Build history of the part. All positions in model axes, mm. A direction names the side the tool comes from. Give positions to 0.01 mm unless a question says otherwise; leave off trailing zeros. Order: outer loops, then holes, each group sorted by start corner. A loop starts at its lowest first (then second) coordinate and runs counter-clockwise, first axis right, second up. Notation, with made-up numbers: (5, 49.25) - (14, 49.25) arc R11 ccw to (14, 54.25) - close; hole circle Ø6 at (85.5, -39.5). An arc over 180 degrees is marked (long way). Use a Markdown table: item, result. Add a question column.
(1) Slice it at A-A (y = 6). Write the cut outline in (x, z).
(2) Flat gauge pins, fed straight in: pin 1 (15 mm diameter, centred on x = -20, z = 1.5, fed in from +Y); pin 2 (6 mm diameter, centred on y = 36.5, z = 20.5, fed in from -X); pin 3 (12 mm diameter, centred on x = -31, y = 32, fed in from +Z). Where does each tip first touch, or does it go through?
(3) Slice it at B-B (x = 0). Write the cut outline in (y, z), then the cut area to 3 significant figures.
(4) Slice it at C-C (y = 60). Write the cut outline in (x, z).
(5) Slice it at D-D (z = 21.5). Write the cut outline in (x, y), then the cut area to 3 significant figures.
(6) Wall check: line 1 (X direction, y = 5.5, z = -4.5); line 2 (Z direction, x = 30, y = 4); line 3 (Y direction, x = -0.5, z = 8). Give the ranges that are in metal, low to high.
(7) Which spindle directions (+Z, -Z, +X, -X, +Y, -Y) get a long thin tool onto all of the face, cutting with end or side? Do faces 1 (the face through (45.49, 5.07, -15.72)), 2 (the face through (-1, 10, -5)). Say none if no direction does.
(8) Mould opens along Z. For faces 3 (the face through (1, 38, 10)), 4 (the face through (50, 5, 8)), 5 (the face through (-25.105, 4.92, -5.215)) say: +Z half, -Z half, draft (parallel to the pull), parting line (faces both ways), or undercut.
from build123d import *

# Parameters (mm, degrees)
CROQUIS1_W                           = 100
CROQUIS1_H                           = 40
SALIENTE_EXTRUIR1_DEPTH              = 10
CROQUIS2_R                           = 8
SALIENTE_EXTRUIR2_DEPTH              = 10
SALIENTE_EXTRUIR3_START              = 5
CROQUIS3_R                           = 20
CROQUIS3_R_2                         = 8
SALIENTE_EXTRUIR3_DEPTH              = 5
F_9_8_9_8_DIAMETER_HOLE1_D           = 9.8
F_9_8_9_8_DIAMETER_HOLE1_CSINK_D     = 9.85
F_9_8_9_8_DIAMETER_HOLE1_CSINK_ANGLE = 100
F_10_0_10_DIAMETER_HOLE1_D           = 10
F_10_0_10_DIAMETER_HOLE1_CSINK_D     = 10.05
F_10_0_10_DIAMETER_HOLE1_CSINK_ANGLE = 100
REDONDEO1_R                          = 15


with BuildPart() as part:
    # Croquis1 → Saliente-Extruir1 (new body)
    with BuildSketch(Plane(origin=(0, 0, 0), x_dir=(1, 0, 0), z_dir=(0, 1, 0))):
        Rectangle(CROQUIS1_W, CROQUIS1_H)
    extrude(amount=SALIENTE_EXTRUIR1_DEPTH)

    # Croquis2 → Saliente-Extruir2 (add)
    with BuildSketch(Plane.XY.offset(20)):
        with BuildLine():
            Line((-50, 10), (-17.564659966, 69.564659966))
            ThreePointArc((-17.564659966, 69.564659966), (0, 80), (17.564659966, 69.564659966))
            Line((17.564659966, 69.564659966), (50, 10))
            Line((50, 10), (-50, 10))
        make_face()
        with Locations((0, 60)):
            Circle(CROQUIS2_R, mode=Mode.SUBTRACT)
    extrude(amount=-SALIENTE_EXTRUIR2_DEPTH)

    # Croquis3 → Saliente-Extruir3 (add)
    with BuildSketch(Plane.XY.offset(20).offset(SALIENTE_EXTRUIR3_START)):
        with Locations((0, 60)):
            Circle(CROQUIS3_R)
        with Locations((0, 60)):
            Circle(CROQUIS3_R_2, mode=Mode.SUBTRACT)
    extrude(amount=-SALIENTE_EXTRUIR3_DEPTH)

    # Ø9.8 (9.8) Diameter Hole1 (through all)
    with Locations(Plane(origin=(0, 10, 0), x_dir=(1, 0, 0), z_dir=(0, 1, 0))):
        with Locations((-30, 5)):
            CounterSinkHole(F_9_8_9_8_DIAMETER_HOLE1_D / 2, F_9_8_9_8_DIAMETER_HOLE1_CSINK_D / 2, counter_sink_angle=F_9_8_9_8_DIAMETER_HOLE1_CSINK_ANGLE)

    # Ø10.0 (10) Diameter Hole1 (through all)
    with Locations(Plane(origin=(0, 10, 0), x_dir=(1, 0, 0), z_dir=(0, 1, 0))):
        with Locations((30, 5)):
            CounterSinkHole(F_10_0_10_DIAMETER_HOLE1_D / 2, F_10_0_10_DIAMETER_HOLE1_CSINK_D / 2, counter_sink_angle=F_10_0_10_DIAMETER_HOLE1_CSINK_ANGLE)

    # Redondeo1
    redondeo1_edges = [part.edges().sort_by_distance(p)[0] for p in [
        (-50, 5, -20),
        (50, 5, -20),
    ]]
    fillet(redondeo1_edges, radius=REDONDEO1_R)


solid = part.part
Solution:
| question | item | result |
|---|---|---|
| 1 | outline | (-50, -5) arc R15 ccw to (-35, -20) - (35, -20) arc R15 ccw to (50, -5) - (50, 20) - (-50, 20) - close; hole circle Ø9.8 at (-30, -5); hole circle Ø10 at (30, -5) |
| 2 | pin 1 | y = 10 |
| 2 | pin 2 | x = -37.18 |
| 2 | pin 3 | z = 20 |
| 3 | outline | (0, -20) - (10, -20) - (10, 10) - (52, 10) - (52, 25) - (40, 25) - (40, 20) - (0, 20) - close; (68, 10) - (80, 10) - (80, 25) - (68, 25) - close |
| 3 | area | 1,060 mm2 |
| 4 | outline | (-22.77, 10) - (-8, 10) - (-8, 25) - (-20, 25) - (-20, 20) - (-22.77, 20) - close; (8, 10) - (22.77, 10) - (22.77, 20) - (20, 20) - (20, 25) - (8, 25) - close |
| 5 | outline | circle Ø40 at (0, 60); hole circle Ø16 at (0, 60) |
| 5 | area | 1,060 mm2 |
| 6 | line 1 | -50 to -34.87, -25.13 to 25.03, 34.97 to 50 |
| 6 | line 2 | -20 to -10, 0 to 20 |
| 6 | line 3 | 0 to 10 |
| 7 | face 1 | -Z, +X, +Y, -Y |
| 7 | face 2 | -Z, +X, -X, +Y |
| 8 | face 3 | -Z half |
| 8 | face 4 | draft |
| 8 | face 5 | undercut |
